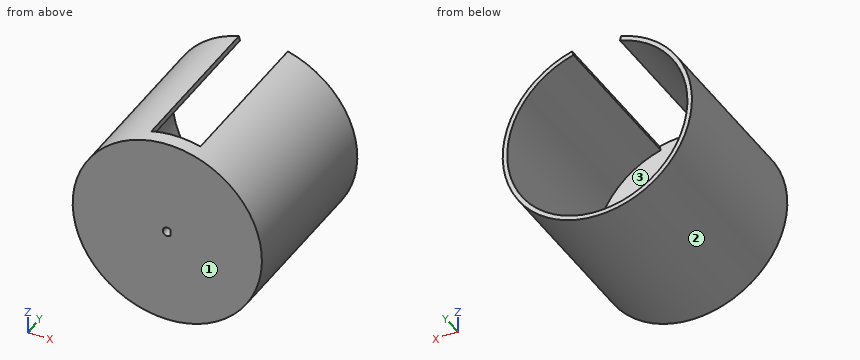
```python
from build123d import *

# Parameters (mm, degrees)
ESQUISSE1_W             = 31.5
ESQUISSE1_H             = 60
ENL_V_START             = -55
ESQUISSE2_R             = 30
ENL_V_MAT_EXTRU_4_DEPTH = 55
ENL_V_MAT_EXTRU_7_DEPTH = 4


with BuildPart() as part:
    # Esquisse1 → Révolution1 (revolve)
    with BuildSketch(Plane.XY, mode=Mode.PRIVATE) as r_volution1_sk:
        with Locations((15.75, 30)):
            Rectangle(ESQUISSE1_W, ESQUISSE1_H)
    revolve(r_volution1_sk.sketch.rotate(Axis((0, 0, 0), (0, 1, 0)), 90), axis=Axis((0, 0, 0), (0, 1, 0)))

    # Esquisse2 → Enlèv. mat.-Extru.4 (cut)
    with BuildSketch(Plane(origin=(0, 60, 0), x_dir=(1, 0, 0), z_dir=(0, 1, 0)).offset(ENL_V_START)):
        Circle(ESQUISSE2_R)
        with BuildLine():
            Line((-7.923821592, -30.487096473), (0, 0))
            Line((0, 0), (8.381317443, -30.36451083))
            ThreePointArc((8.381317443, -30.36451083), (0.236817278, -31.49910979), (-7.923821592, -30.487096473))
        make_face()
    extrude(amount=ENL_V_MAT_EXTRU_4_DEPTH, mode=Mode.SUBTRACT)

    # Esquisse4 → Enlèv. mat.-Extru.7 (cut)
    with BuildSketch(Plane(origin=(0, 0, 0), x_dir=(-1, 0, 0), z_dir=(0, -1, 0))):
        with BuildLine():
            Line((-1, 1.118033989), (-1, -1.118033989))
            ThreePointArc((-1, -1.118033989), (0.612372436, -1.369306394), (1.5, 0))
            ThreePointArc((1.5, 0), (0.612372436, 1.369306394), (-1, 1.118033989))
        make_face()
    extrude(amount=-ENL_V_MAT_EXTRU_7_DEPTH, mode=Mode.SUBTRACT)


solid = part.part
```
Geometry check sheet. Reference: the model listing, model coordinates, mm. Face numbers are marked on the shaded views. Coordinates: 2 decimals unless noted, no trailing zeros. Order: outer loops, then holes, each group sorted by start corner. A loop starts at its lowest first (then second) coordinate and runs counter-clockwise, first axis right, second up.
Item 1: Section check C-C (y = 20). Enter the section's corners in (x, z).
Item 2: Scan lines: line 1 along X through (y, z) = (24.5, 0); line 2 along Y through (x, z) = (-27, -12); line 3 along Z through (x, y) = (-14, 16). Record each from-to range of solid material in increasing order.
Item 3: Section check D-D (x = -15). Enter the section's corners in (y, z), plus the area to 3 significant figures.
Item 4: Section check A-A (x = 0). Enter the section's corners in (y, z), plus the area to 4 significant figures.
Item 5: Mould release check, pull along X, two halves, no side actions. Record for the marked faces 1, 2 and 3: released by +X, released by -X, zero draft, split by the parting line, or undercut.
Item 6: Depth check by flat-ended pin: pin 1 (1.5 mm diameter, centred on y = 15.5, z = 10.5, fed in from +X); pin 2 (6 mm diameter, centred on y = 45, z = -21, fed in from +X); pin 3 (3 mm diameter, centred on x = -1, z = -0.5, fed in from -Y); pin 4 (10 mm diameter, centred on x = 23, y = 37, fed in from -Z). Enter the tip coordinate at first touch or a pass-through.
Item 7: Section check B-B (z = -3.5). Enter the section's corners in (x, y).
Check sheet entries:
1. outline: (-7.92, 30.49) arc R31.5 ccw (long way) to (8.38, 30.36) - (7.98, 28.92) arc R30 cw (long way) to (-7.55, 29.04) - close
2. line 1: x = -31.5 to -30, 30 to 31.5
2. line 2: y = 0 to 5
2. line 3: z = -28.22 to -26.53, 26.53 to 28.22
3. outline: (0, -27.7) - (60, -27.7) - (60, -25.98) - (5, -25.98) - (5, 25.98) - (60, 25.98) - (60, 27.7) - (0, 27.7) - close
3. area: 466 mm2
4. outline: (0, -31.5) - (60, -31.5) - (60, -30) - (5, -30) - (5, 31.5) - (0, 31.5) - (0, 1.5) - (4, 1.5) - (4, -1.5) - (0, -1.5) - close
4. area: 385.5 mm2
5. face 1: zero draft
5. face 2: split by the parting line
5. face 3: undercut
6. pin 1: stops at x = 29.95
6. pin 2: stops at x = 25.85
6. pin 3: stops at y = 0
6. pin 4: stops at z = -25.85
7. outline: (-31.3, 0) - (31.3, 0) - (31.3, 60) - (29.8, 60) - (29.8, 5) - (-29.8, 5) - (-29.8, 60) - (-31.3, 60) - close
